from build123d import *

# Parameters (mm, degrees)
SKETCH1_R           = 4
BOSS_EXTRUDE1_DEPTH = 2.5
BOSS_EXTRUDE5_DEPTH = 2
SKETCH10_R          = 1
BOSS_EXTRUDE6_DEPTH = 2
FILLET1_R           = 5
SKETCH11_R          = 1.25
CUT_EXTRUDE1_DEPTH  = 12


with BuildPart() as part:
    # Sketch1 → Boss-Extrude1 (new body)
    with BuildSketch(Plane(origin=(0, 0, 0), x_dir=(1, 0, 0), z_dir=(0, 1, 0))):
        with Locations((-36.385139863, -3.349743035)):
            Circle(SKETCH1_R)
        with BuildLine():
            Line((-36.385139863, -0.349743035), (-36.427751557, -0.423548653))
            ThreePointArc((-36.427751557, -0.423548653), (-36.842946049, -0.459268538), (-37.248857528, -0.553599062))
            Line((-37.248857528, -0.553599062), (-37.312190847, -0.496573486))
            Line((-37.312190847, -0.496573486), (-37.329909785, -0.579934537))
            ThreePointArc((-37.329909785, -0.579934537), (-37.713745161, -0.742208321), (-38.070640183, -0.957355526))
            Line((-38.070640183, -0.957355526), (-38.14849562, -0.922692052))
            Line((-38.14849562, -0.922692052), (-38.139587351, -1.007448576))
            ThreePointArc((-38.139587351, -1.007448576), (-38.454491129, -1.28039177), (-38.727434323, -1.595295548))
            Line((-38.727434323, -1.595295548), (-38.812190847, -1.586387278))
            Line((-38.812190847, -1.586387278), (-38.777527372, -1.664242716))
            ThreePointArc((-38.777527372, -1.664242716), (-38.992674577, -2.021137738), (-39.154948361, -2.404973114))
            Line((-39.154948361, -2.404973114), (-39.238309412, -2.422692052))
            Line((-39.238309412, -2.422692052), (-39.181283836, -2.486025371))
            ThreePointArc((-39.181283836, -2.486025371), (-39.27561436, -2.89193685), (-39.311334246, -3.307131342))
            Line((-39.311334246, -3.307131342), (-39.385139863, -3.349743035))
            Line((-39.385139863, -3.349743035), (-39.311334246, -3.392354728))
            ThreePointArc((-39.311334246, -3.392354728), (-39.27561436, -3.80754922), (-39.181283836, -4.2134607))
            Line((-39.181283836, -4.2134607), (-39.238309412, -4.276794018))
            Line((-39.238309412, -4.276794018), (-39.154948361, -4.294512957))
            ThreePointArc((-39.154948361, -4.294512957), (-38.992674577, -4.678348332), (-38.777527372, -5.035243354))
            Line((-38.777527372, -5.035243354), (-38.812190847, -5.113098792))
            Line((-38.812190847, -5.113098792), (-38.727434323, -5.104190522))
            ThreePointArc((-38.727434323, -5.104190522), (-38.454491129, -5.419094301), (-38.139587351, -5.692037494))
            Line((-38.139587351, -5.692037494), (-38.14849562, -5.776794018))
            Line((-38.14849562, -5.776794018), (-38.070640183, -5.742130544))
            ThreePointArc((-38.070640183, -5.742130544), (-37.713745161, -5.957277749), (-37.329909785, -6.119551533))
            Line((-37.329909785, -6.119551533), (-37.312190847, -6.202912584))
            Line((-37.312190847, -6.202912584), (-37.248857528, -6.145887008))
            ThreePointArc((-37.248857528, -6.145887008), (-36.842946049, -6.240217532), (-36.427751557, -6.275937417))
            Line((-36.427751557, -6.275937417), (-36.385139863, -6.349743035))
            Line((-36.385139863, -6.349743035), (-36.34252817, -6.275937417))
            ThreePointArc((-36.34252817, -6.275937417), (-35.927333678, -6.240217532), (-35.521422199, -6.145887008))
            Line((-35.521422199, -6.145887008), (-35.45808888, -6.202912584))
            Line((-35.45808888, -6.202912584), (-35.440369942, -6.119551533))
            ThreePointArc((-35.440369942, -6.119551533), (-35.056534566, -5.957277749), (-34.699639544, -5.742130544))
            Line((-34.699639544, -5.742130544), (-34.621784107, -5.776794018))
            Line((-34.621784107, -5.776794018), (-34.630692376, -5.692037494))
            ThreePointArc((-34.630692376, -5.692037494), (-34.315788598, -5.419094301), (-34.042845404, -5.104190522))
            Line((-34.042845404, -5.104190522), (-33.95808888, -5.113098792))
            Line((-33.95808888, -5.113098792), (-33.992752354, -5.035243354))
            ThreePointArc((-33.992752354, -5.035243354), (-33.77760515, -4.678348332), (-33.615331365, -4.294512957))
            Line((-33.615331365, -4.294512957), (-33.531970315, -4.276794018))
            Line((-33.531970315, -4.276794018), (-33.588995891, -4.2134607))
            ThreePointArc((-33.588995891, -4.2134607), (-33.494665367, -3.80754922), (-33.458945481, -3.392354728))
            Line((-33.458945481, -3.392354728), (-33.385139863, -3.349743035))
            Line((-33.385139863, -3.349743035), (-33.458945481, -3.307131342))
            ThreePointArc((-33.458945481, -3.307131342), (-33.494665367, -2.89193685), (-33.588995891, -2.486025371))
            Line((-33.588995891, -2.486025371), (-33.531970315, -2.422692052))
            Line((-33.531970315, -2.422692052), (-33.615331365, -2.404973114))
            ThreePointArc((-33.615331365, -2.404973114), (-33.77760515, -2.021137738), (-33.992752354, -1.664242716))
            Line((-33.992752354, -1.664242716), (-33.95808888, -1.586387278))
            Line((-33.95808888, -1.586387278), (-34.042845404, -1.595295548))
            ThreePointArc((-34.042845404, -1.595295548), (-34.315788598, -1.28039177), (-34.630692376, -1.007448576))
            Line((-34.630692376, -1.007448576), (-34.621784107, -0.922692052))
            Line((-34.621784107, -0.922692052), (-34.699639544, -0.957355526))
            ThreePointArc((-34.699639544, -0.957355526), (-35.056534566, -0.742208321), (-35.440369942, -0.579934537))
            Line((-35.440369942, -0.579934537), (-35.45808888, -0.496573486))
            Line((-35.45808888, -0.496573486), (-35.521422199, -0.553599062))
            ThreePointArc((-35.521422199, -0.553599062), (-35.927333678, -0.459268538), (-36.34252817, -0.423548653))
            Line((-36.34252817, -0.423548653), (-36.385139863, -0.349743035))
        make_face(mode=Mode.SUBTRACT)
    extrude(amount=BOSS_EXTRUDE1_DEPTH)

    # Sketch2 → Boss-Extrude5 (add)
    with BuildSketch(Plane.XZ):
        with BuildLine():
            ThreePointArc((-40.385139863, 3.349743035), (-36.385139863, -0.650256965), (-32.385139863, 3.349743035))
            Line((-32.385139863, 3.349743035), (-32.385139863, 13.349743035))
            Line((-32.385139863, 13.349743035), (-40.385139863, 13.349743035))
            Line((-40.385139863, 13.349743035), (-40.385139863, 3.349743035))
        make_face()
    extrude(amount=BOSS_EXTRUDE5_DEPTH)

    # Sketch10 → Boss-Extrude6 (add)
    with BuildSketch(Plane.XY.offset(13.349743035)):
        Polygon((-13.885139863, 0), (-58.885139863, 0), (-58.885139863, -20), (-45.380774313, -20), (-45.380774313, -15.439425839), (-27.389505414, -16), (-27.389505414, -20), (-13.885139863, -20), align=None)
        with Locations((-56.885139863, -18)):
            Circle(SKETCH10_R, mode=Mode.SUBTRACT)
        with Locations((-15.885139863, -18)):
            Circle(SKETCH10_R, mode=Mode.SUBTRACT)
        with Locations((-56.885139863, -2)):
            Circle(SKETCH10_R, mode=Mode.SUBTRACT)
        with Locations((-15.885139863, -2)):
            Circle(SKETCH10_R, mode=Mode.SUBTRACT)
    extrude(amount=BOSS_EXTRUDE6_DEPTH)

    # Fillet1
    fillet1_edges = [part.edges().sort_by_distance(p)[0] for p in [
        (-36.385139863, -2, 13.349743035),
    ]]
    fillet(fillet1_edges, radius=FILLET1_R)

    # Sketch11 → Cut-Extrude1 (cut)
    with BuildSketch(Plane.XZ.offset(2)):
        with Locations((-36.385139863, 3.349743035)):
            Circle(SKETCH11_R)
    extrude(amount=-CUT_EXTRUDE1_DEPTH, mode=Mode.SUBTRACT)


solid = part.part
Geometry check sheet. Reference: the model listing, model coordinates, mm. A direction names the side the tool comes from. Give positions to 0.01 mm unless a question says otherwise; leave off trailing zeros. Write each loop counter-clockwise with the first axis right and the second up, starting at its lowest first coordinate (ties: lowest second). Pieces come first, ordered by that corner, then holes.
1) Cross-section at B-B (x = -21). Record the boundary of the cut face in (y, z), plus the area to 3 significant figures.
Values follow:
outline: (-20, 13.35) - (0, 13.35) - (0, 15.35) - (-20, 15.35) - close
area: 40.0 mm2
2) Cross-section at A-A (y = -18). Record the boundary of the cut face in (x, z).
Values follow:
outline: (-58.89, 13.35) - (-57.89, 13.35) - (-57.89, 15.35) - (-58.89, 15.35) - close; (-55.89, 13.35) - (-45.38, 13.35) - (-45.38, 15.35) - (-55.89, 15.35) - close; (-27.39, 13.35) - (-16.89, 13.35) - (-16.89, 15.35) - (-27.39, 15.35) - close; (-14.89, 13.35) - (-13.89, 13.35) - (-13.89, 15.35) - (-14.89, 15.35) - close
3) Thickness scan on line 1 (Z direction, x = -40.5, y = -8); line 2 (X direction, y = -1.25, z = 8.5); line 3 (Y direction, x = -34.5, z = 5). Record the ranges inside material, lowest first.
Values follow:
line 1: z = 13.35 to 15.35
line 2: x = -40.39 to -32.39
line 3: y = -2 to 0
4) Go/stop test with flat-tipped pins: pin 1 Ø7.5 at (y, z) = (-5, 10) entering from -X; pin 2 Ø1.2 at (x, y) = (-15.89, -18) entering from -Z; pin 3 Ø1.5 at (x, z) = (-38, 1) entering from -Y; pin 4 Ø4 at (x, y) = (-38, -17.5) entering from -Z. Record where each tip stops, or that it passes through.
Values follow:
pin 1: stops at x = -58.89
pin 2: passes through
pin 3: stops at y = -2
pin 4: stops at z = 13.35
5) Set-up check for faces 1 (the face through (-36, -2, 5)), 2 (the face through (-16.884, -1.956, 14.336)), 3 (the face through (-35.92, 1.23, 0.46)): record each of +Z, -Z, +X, -X, +Y, -Y from which the full face is reachable in a straight line by a thin tool's end or side.
Values follow:
face 1: -Z, +X, -X, -Y
face 2: +Z, -Z
face 3: +Y
6) Cross-section at C-C (z = 9.75). Record the boundary of the cut face in (x, y).
Values follow:
outline: (-40.39, -2.2) - (-32.39, -2.2) - (-32.39, 0) - (-40.39, 0) - close
7) Release check for a two-part mould opening along X. For faces 4 (the face through (-58.885, -10, 14)), 5 (the face through (-33.494, 1.232, 2.898)), 6 (the face through (-36, 0, 13)), 7 (the face through (-32.385, -1, 8)) record: released by +X, released by -X, zero draft, split by the parting line, or undercut.
Values follow:
face 4: released by -X
face 5: undercut
face 6: zero draft
face 7: released by +X
